Geometry: final body of the model. Coordinates: model frame, mm. Face numbers are marked on the shaded views. A direction names the side the tool comes from. Coordinates: 2 decimals unless noted, no trailing zeros. Loops run counter-clockwise (first coordinate to the right, second up) from the corner with the lowest first, then second, coordinate; pieces in that order, holes last. Notation, with made-up numbers: M 14.5,-38 L 45.5,-38 A17 ccw 45.5,-15 Z; hole C 7,-38 d8. An arc over 180 degrees is marked long. Write each question's results on one line, items separated by ' | '. Start each with the question number.
from build123d import *

# Parameters (mm, degrees)
SKETCH1_R           = 1.7
BOSS_EXTRUDE1_DEPTH = 8
CUT_EXTRUDE1_DEPTH  = 2.5
CUT_EXTRUDE2_DEPTH  = 4.3


with BuildPart() as part:
    # Sketch1 → Boss-Extrude1 (new body)
    with BuildSketch(Plane.XY):
        with BuildLine():
            Line((-16, 5), (16, 5))
            ThreePointArc((16, 5), (21, 0), (16, -5))
            Line((16, -5), (-16, -5))
            ThreePointArc((-16, -5), (-21, 0), (-16, 5))
        make_face()
        with Locations((-14.2222, 0)):
            Circle(SKETCH1_R, mode=Mode.SUBTRACT)
        with Locations((16, 0)):
            Circle(SKETCH1_R, mode=Mode.SUBTRACT)
    extrude(amount=BOSS_EXTRUDE1_DEPTH)

    # Sketch3 → Cut-Extrude1 (cut)
    with BuildSketch(Plane.XY.offset(8)):
        with BuildLine():
            Line((-20.2222, 3.15), (-14.2222, 3.15))
            ThreePointArc((-14.2222, 3.15), (-11.0722, 0), (-14.2222, -3.15))
            Line((-14.2222, -3.15), (-20.2222, -3.15))
            ThreePointArc((-20.2222, -3.15), (-23.3722, 0), (-20.2222, 3.15))
        make_face()
    extrude(amount=-CUT_EXTRUDE1_DEPTH, mode=Mode.SUBTRACT)

    # Sketch4 → Cut-Extrude2 (cut)
    with BuildSketch(Plane.XY.offset(5.5)):
        with BuildLine():
            Line((-21, 4.15), (-14.2222, 4.15))
            ThreePointArc((-14.2222, 4.15), (-10.0722, 0), (-14.2222, -4.15))
            Line((-14.2222, -4.15), (-21, -4.15))
            ThreePointArc((-21, -4.15), (-25.15, 0), (-21, 4.15))
        make_face()
    extrude(amount=-CUT_EXTRUDE2_DEPTH, mode=Mode.SUBTRACT)


solid = part.part
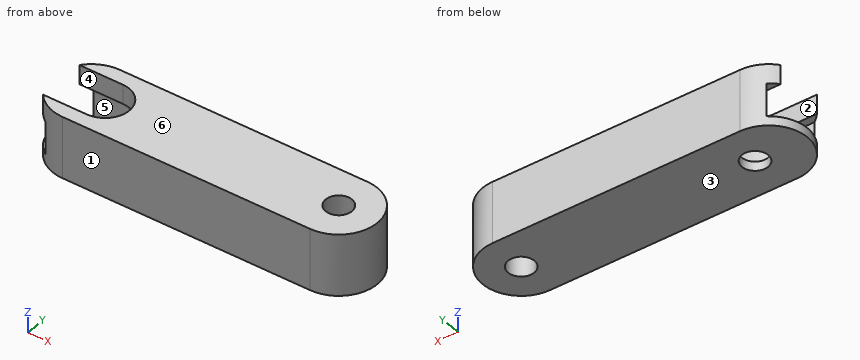
Item 1: Section A-A, the plane y = 0. Return loops of the section in (x, z).
Item 2: Contact query for flat-ended pins moving along their axis: P1, Ø3, axis at y = 2.5, z = 1.5, coming from the -X side; P2, Ø2.5, axis at x = -14, y = -1, coming from the +Z side; P3, Ø1.5, axis at y = -1, z = 4.5, coming from the -X side; P4, Ø2, axis at x = -14.22, y = 0, coming from the +Z side. Output: stop coordinate, or through.
Item 3: Section C-C, the plane x = -13. Return loops of the section in (y, z).
Item 4: Section D-D, the plane z = 3.75. Return loops of the section in (x, y).
Item 5: Ray query, L1, parallel to Y at x = 16, z = 3.25; L2, parallel to Z at x = -15, y = -1.75; L3, parallel to Y at x = -13.5, z = 2.5. Return the intervals inside material, ascending. Write a range as [from, to].
Item 6: Pull-direction query (Y, two-part tool) for the marked faces 1, 2 and 3; classes: released by +Y, released by -Y, zero draft, split by the parting line, or undercut.
Item 7: Section B-B, the plane z = 6.75. Return loops of the section in (x, y).
Item 8: Set-up query: the marked faces 4, 5 and 6. Return all of +Z, -Z, +X, -X, +Y, -Y with unobstructed straight access to the full face (end or side cutting, diameter ignored); none if empty.
Solutions:
1) outline: M -21,0 L -15.92,0 L -15.92,1.2 L -21,1.2 Z; M -12.52,0 L 14.3,0 L 14.3,8 L -11.07,8 L -11.07,5.5 L -10.07,5.5 L -10.07,1.2 L -12.52,1.2 Z; M 17.7,0 L 21,0 L 21,8 L 17.7,8 Z
2) P1: stops at x = -20.89 | P2: stops at z = 1.2 | P3: stops at x = -10.46 | P4: passes through
3) outline: M -5,0 L -1.18,0 L -1.18,1.2 L -3.97,1.2 L -3.97,5.5 L -2.9,5.5 L -2.9,8 L -5,8 Z; M 1.18,0 L 5,0 L 5,8 L 2.9,8 L 2.9,5.5 L 3.97,5.5 L 3.97,1.2 L 1.18,1.2 Z
4) outline: M -18.79,-4.15 A5 ccw -16,-5 L 16,-5 A5 ccw 16,5 L -16,5 A5 ccw -18.79,4.15 L -14.22,4.15 A4.15 cw -14.22,-4.15 Z; hole C 16,0 d3.4
5) L1: y = [-5, -1.7], [1.7, 5] | L2: z = [0, 1.2] | L3: y = [-5, -4.09], [4.09, 5]
6) face 1: released by -Y | face 2: undercut | face 3: zero draft
7) outline: M -19.88,-3.15 A5 ccw -16,-5 L 16,-5 A5 ccw 16,5 L -16,5 A5 ccw -19.88,3.15 L -14.22,3.15 A3.15 cw -14.22,-3.15 Z; hole C 16,0 d3.4
8) face 4: +Z, -X | face 5: -X | face 6: +Z, +X, -X, +Y, -Y
